The figure shows three views and two pictorial views of one solid part (mm, origin at its lowest corner). Answer the questions. Coordinates: 2 decimals unless noted, no trailing zeros. Order: outer loops, then holes, each group sorted by start corner. A loop starts at its lowest first (then second) coordinate and runs counter-clockwise, first axis right, second up. Notation, with made-up numbers: M 2,-34 L 57,-34 A19 cw 57,-29 Z; hole C -18,74.5 d2. An arc over 180 degrees is marked long. Answer in a Markdown table with one row per item. Add a question column.
Item 1: The part is cut by section B-B (z = 7.5). Write down the section's boundary in (x, y), then the cut area to 3 significant figures.
Item 2: A flat-ended cylindrical pin translates along its axis: pin 1 Ø4 at (x, z) = (7.5, 7.5) entering from -Y. Find the tip coordinate at first contact, or state that the pin passes through.
Item 3: The part is cut by section A-A (x = 7.5). Write down the section's boundary in (y, z).
Item 4: The mould has two halves that part along X. Classify the marked faces 1, 2 and 3: released by +X, released by -X, zero draft, split by the parting line, or undercut.
Item 5: The part is cut by section C-C (y = 3.4). Write down the section's boundary in (x, z).
Item 6: Consider line 1 (Z direction, x = 7.5, y = 1.7); line 2 (X direction, y = 2.95, z = 5.75); line 3 (X direction, y = 3.25, z = 8.75). Determine where each line is inside the solid, lowest interval first. Write a range as from..to.
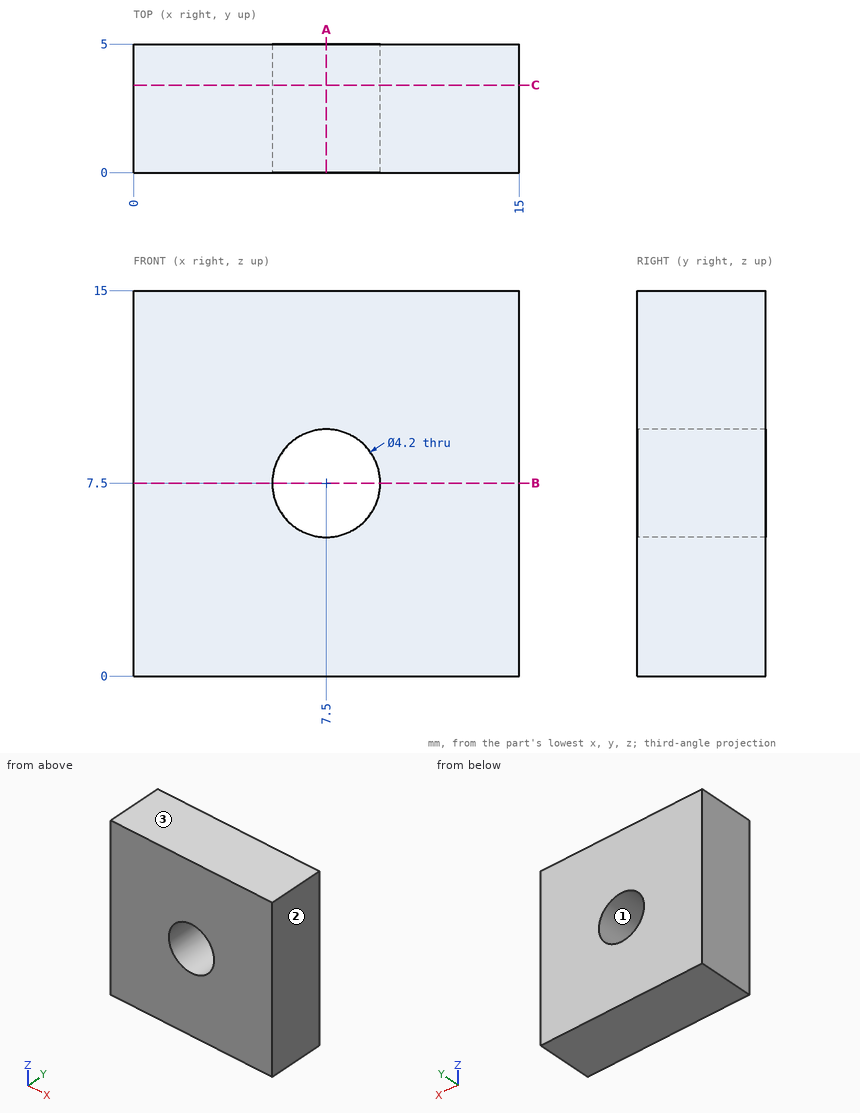
Reply:
| question | item | result |
|---|---|---|
| 1 | outline | M 0,0 L 5.4,0 L 5.4,5 L 0,5 Z; M 9.6,0 L 15,0 L 15,5 L 9.6,5 Z |
| 1 | area | 54.0 mm2 |
| 2 | pin 1 | passes through |
| 3 | outline | M 0,0 L 5,0 L 5,5.4 L 0,5.4 Z; M 0,9.6 L 5,9.6 L 5,15 L 0,15 Z |
| 4 | face 1 | undercut |
| 4 | face 2 | released by +X |
| 4 | face 3 | zero draft |
| 5 | outline | M 0,0 L 15,0 L 15,15 L 0,15 Z; hole C 7.5,7.5 d4.2 |
| 6 | line 1 | z = 0..5.4, 9.6..15 |
| 6 | line 2 | x = 0..6.34, 8.66..15 |
| 6 | line 3 | x = 0..5.81, 9.19..15 |
